The model under review builds one solid part; all positions refer to its coordinate system, in mm. A direction names the side the tool comes from. Round coordinates to 2 decimals unless told otherwise and drop trailing zeros. Loops run counter-clockwise (first coordinate to the right, second up) from the corner with the lowest first, then second, coordinate; pieces in that order, holes last. Notation, with made-up numbers: M 58,45 L 74,45 A18 ccw 74,49 Z; hole C -5.75,7.25 d9. An arc over 180 degrees is marked long. One line per question, with ' | ' between items.
from build123d import *

# Parameters (mm, degrees)
BOSS_EXTRUDE1_DEPTH     = 20
BOSS_EXTRUDE2_DEPTH     = 15
SKETCH1_4_R             = 10
BOSS_EXTRUDE3_DEPTH     = 15
BOSS_EXTRUDE4_START     = -20
SKETCH1_5_R             = 10
BOSS_EXTRUDE4_DEPTH     = 20
FILLET1_R               = 20
SKETCH2_W               = 40
SKETCH2_H               = 10
BOSS_EXTRUDE5_DEPTH     = 10
SKETCH3_R               = 10
BOSS_EXTRUDE6_DEPTH     = 10
CUT_EXTRUDE1_DEPTH      = 107.066017178
CUT_EXTRUDE1_DEPTH_BACK = 107.066017178
SKETCH4_R               = 10


with BuildPart() as part:
    # Sketch1 → Boss-Extrude1 (new body)
    with BuildSketch(Plane.YZ):
        Polygon((20, -20), (-20, -20), (-80, -20), (-80, -30), (80, -30), (80, -20), align=None)
    extrude(amount=-BOSS_EXTRUDE1_DEPTH)

    # Sketch1_3 → Boss-Extrude2 (add)
    with BuildSketch(Plane.YZ):
        Polygon((20, -20), (-20, -20), (-80, -20), (-80, -30), (80, -30), (80, -20), align=None)
    extrude(amount=BOSS_EXTRUDE2_DEPTH)

    # Sketch1_4 → Boss-Extrude3 (add)
    with BuildSketch(Plane.YZ):
        with BuildLine():
            Line((20, -20), (20, 0))
            ThreePointArc((20, 0), (0, 20), (-20, 0))
            Line((-20, 0), (-20, -20))
            Line((-20, -20), (20, -20))
        make_face()
        with Locations(Location((0, 0, 0), (0, 0, 270))):
            Circle(SKETCH1_4_R, mode=Mode.SUBTRACT)
    extrude(amount=BOSS_EXTRUDE3_DEPTH)

    # Sketch1_5 → Boss-Extrude4 (add)
    with BuildSketch(Plane.YZ.offset(BOSS_EXTRUDE4_START)):
        with BuildLine():
            Line((20, -20), (20, 0))
            ThreePointArc((20, 0), (0, 20), (-20, 0))
            Line((-20, 0), (-20, -20))
            Line((-20, -20), (20, -20))
        make_face()
        with Locations(Location((0, 0, 0), (0, 0, 270))):
            Circle(SKETCH1_5_R, mode=Mode.SUBTRACT)
    extrude(amount=BOSS_EXTRUDE4_DEPTH)

    # Fillet1
    fillet1_edges = [part.edges().sort_by_distance(p)[0] for p in [
        (-20, 80, -25),
        (-20, -80, -25),
    ]]
    fillet(fillet1_edges, radius=FILLET1_R)

    # Sketch2 → Boss-Extrude5 (add)
    with BuildSketch(Plane.YZ.offset(15)):
        with Locations((-60, -25)):
            Rectangle(SKETCH2_W, SKETCH2_H)
        with Locations((60, -25)):
            Rectangle(SKETCH2_W, SKETCH2_H)
    extrude(amount=BOSS_EXTRUDE5_DEPTH)

    # Sketch3 → Boss-Extrude6 (add)
    # profile 1 of 2: a face of its own
    with BuildSketch(Plane.YZ.offset(25)):
        with BuildLine():
            Line((-80, -20), (-40, -20))
            Line((-40, -20), (-40, -45))
            ThreePointArc((-40, -45), (-60, -65), (-80, -45))
            Line((-80, -45), (-80, -20))
        make_face()
        with Locations(Location((-60, -45, 0), (0, 0, 270))):
            Circle(SKETCH3_R, mode=Mode.SUBTRACT)
    # profile 2 of 2: a face of its own
    with BuildSketch(Plane.YZ.offset(25)):
        with BuildLine():
            Line((80, -45), (80, -20))
            Line((80, -20), (40, -20))
            Line((40, -20), (40, -45))
            ThreePointArc((40, -45), (60, -65), (80, -45))
        make_face()
        with Locations(Location((60, -45, 0), (0, 0, 90))):
            Circle(SKETCH3_R, mode=Mode.SUBTRACT)
    extrude(amount=-BOSS_EXTRUDE6_DEPTH)

    # Sketch4 → Cut-Extrude1 (cut, two sides: drawn at the far end of the back side and taken through both)
    with BuildSketch(Plane(origin=(0, 0, 0), x_dir=(0, 1, 0), z_dir=(0, 0, 1)).offset(-CUT_EXTRUDE1_DEPTH_BACK)):
        with Locations(Location((-60, 0, 0), (0, 0, 90))):
            Circle(SKETCH4_R)
        with Locations(Location((60, 0, 0), (0, 0, 90))):
            Circle(SKETCH4_R)
    extrude(amount=CUT_EXTRUDE1_DEPTH + CUT_EXTRUDE1_DEPTH_BACK, mode=Mode.SUBTRACT)


solid = part.part
1) Add section A-A on x = 18. State the section outline as (y, z) points, then the cut area to 3 significant figures.
Output values:
outline: M -80,-45 A20 ccw -40,-45 L -40,-20 L -80,-20 Z; M 40,-45 A20 ccw 80,-45 L 80,-20 L 40,-20 Z; hole C -60,-45 d20; hole C 60,-45 d20 | area: 2,630 mm²
2) Add section C-C on z = -22. State the section outline as (x, y) points, then the cut area to 3 significant figures.
Output values:
outline: M -20,-60 A20 ccw 0,-80 L 25,-80 L 25,-40 L 15,-40 L 15,40 L 25,40 L 25,80 L 0,80 A20 ccw -20,60 Z; hole C 0,-60 d20; hole C 0,60 d20 | area: 5,600 mm²
3) Add section B-B on y = 0. State the section outline as (x, z) points.
Output values:
outline: M -20,-30 L 15,-30 L 15,-10 L -20,-10 Z; M -20,10 L 15,10 L 15,20 L -20,20 Z
4) Machinability: for faces 4 (the flat face through (7, 50, -20)), 5 (the flat face through (20, -40, -33)), 6 (the flat face through (15, -64, -55)), which of the approach directions +Z, -Z, +X, -X, +Y, -Y give a long, thin tool a straight path to every point of the face, cutting with its end or side? Answer none if there is none.
Output values:
face 4: +Z, +X, -X, +Y | face 5: +Z, -Z, +X | face 6: -Z, -X, +Y, -Y
5) Mouldability with a two-part tool opening along Y and no side actions: class faces 1 (the flat face through (-3, -1, -30)), 2 (the cylindrical face through (20, 60, -65)), 3 (the flat face through (18, 80, -30)) as +Y half, -Y half, draft (parallel to the pull), parting line (faces both ways), or undercut.
Output values:
face 1: draft | face 2: undercut | face 3: +Y half
6) Add section D-D on x = 5.5. State the section outline as (y, z) points.
Output values:
outline: M -80,-30 L -68.35,-30 L -68.35,-20 L -80,-20 Z; M -51.65,-30 L 51.65,-30 L 51.65,-20 L 20,-20 L 20,0 A20 ccw -20,0 L -20,-20 L -51.65,-20 Z; M 68.35,-30 L 80,-30 L 80,-20 L 68.35,-20 Z; hole C 0,0 d20
7) Insertion check: P1, Ø6, axis at x = 16, z = -9, coming from the -Y side; P2, Ø10.5, axis at y = -67, z = -47, coming from the -X side; P3, Ø10.5, axis at x = 2.5, y = -4, coming from the -Z side. Each pin has a flat end and moves straight along its axis. Give the tip position at first contact, or say it passes through.
Output values:
P1: stops at y = -20 | P2: stops at x = 15 | P3: stops at z = -30
8) For line 1 (Y direction, x = 20.5, z = -45); line 2 (Y direction, x = 0, z = -22.25); line 3 (X direction, y = 15, z = -25.5), list the stretches that pass through material, from the lowest coordinate up.
Output values:
line 1: y = -80 to -70, -50 to -40, 40 to 50, 70 to 80 | line 2: y = -80 to -70, -50 to 50, 70 to 80 | line 3: x = -20 to 15
